Geometry check sheet. Reference: the model listing, model coordinates, mm. Coordinates: 2 decimals unless noted, no trailing zeros. Order: outer loops, then holes, each group sorted by start corner. A loop starts at its lowest first (then second) coordinate and runs counter-clockwise, first axis right, second up. Notation, with made-up numbers: (72.5, 73) - (78.5, 73) arc R14 cw to (78.5, 100) - close; hole circle Ø4 at (7.25, 14.25). An arc over 180 degrees is marked (long way). Put each result on its own line as item: value.
from build123d import *

# Parameters (mm, degrees)
SKETCH1_W                = 304
SKETCH1_H                = 304
BOSS_EXTRUDE1_DEPTH      = 2
SKETCH2_W                = 88
SKETCH2_H                = 15
CUT_EXTRUDE1_DEPTH       = 215.969765316
SKETCH7_W                = 50
SKETCH7_H                = 45
CUT_EXTRUDE2_DEPTH       = 2
FILLET1_R                = 2
F_7_0_7_DIAMETER_HOLE1_D = 7
M5_CLEARANCE_HOLE1_D     = 5.3


with BuildPart() as part:
    # Sketch1 → Boss-Extrude1 (new body)
    with BuildSketch(Plane(origin=(0, 0, 0), x_dir=(1, 0, 0), z_dir=(0, 1, 0))):
        Rectangle(SKETCH1_W, SKETCH1_H)
    extrude(amount=BOSS_EXTRUDE1_DEPTH)

    # Sketch2 → Cut-Extrude1 (cut, through all)
    with BuildSketch(Plane(origin=(0, 2, 0), x_dir=(1, 0, 0), z_dir=(0, 1, 0))):
        with Locations((0, -144.5)):
            Rectangle(SKETCH2_W, SKETCH2_H)
        with BuildLine():
            Line((-152, 100), (-138, 100))
            ThreePointArc((-138, 100), (-128, 110), (-138, 120))
            Line((-138, 120), (-152, 120))
            Line((-152, 120), (-152, 100))
        make_face()
        with BuildLine():
            Line((152, 100), (138, 100))
            ThreePointArc((138, 100), (128, 110), (138, 120))
            Line((138, 120), (152, 120))
            Line((152, 120), (152, 100))
        make_face()
    extrude(amount=-CUT_EXTRUDE1_DEPTH, mode=Mode.SUBTRACT)

    # Sketch7 → Cut-Extrude2 (cut)
    with BuildSketch(Plane.XZ):
        with Locations((0, 114.5)):
            Rectangle(SKETCH7_W, SKETCH7_H)
    extrude(amount=-CUT_EXTRUDE2_DEPTH, mode=Mode.SUBTRACT)

    # Fillet1
    fillet1_edges = [part.edges().sort_by_distance(p)[0] for p in [
        (44, 1, 152),
        (-44, 1, 152),
        (-44, 1, 137),
        (44, 1, 137),
        (-152, 1, -100),
        (-152, 1, -120),
        (152, 1, -120),
        (152, 1, -100),
        (25, 1, 92),
        (25, 1, 137),
        (-25, 1, 137),
        (-25, 1, 92),
        (-152, 1, -152),
        (152, 1, -152),
        (152, 1, 152),
        (-152, 1, 152),
    ]]
    fillet(fillet1_edges, radius=FILLET1_R)

    # Ø7.0 (7) Diameter Hole1 (through all)
    with Locations(Plane(origin=(0, 2, 0), x_dir=(1, 0, 0), z_dir=(0, 1, 0))):
        with Locations((0, -6)):
            Hole(F_7_0_7_DIAMETER_HOLE1_D / 2)

    # M5 Clearance Hole1 (through all)
    with Locations(Plane(origin=(0, 2, 0), x_dir=(1, 0, 0), z_dir=(0, 1, 0))):
        with Locations((-138, 138), (138, 138), (138, -138), (-138, -138), (0, 6)):
            Hole(M5_CLEARANCE_HOLE1_D / 2)


solid = part.part
Q1. Section check B-B on y = 1.55. State how many separate pieces and enclosed holes the cut face has, then the cut area to 3 significant figures.
Answer block:
separate pieces: 1
enclosed holes: 6
area: 87,800 mm^2
Q2. Section check A-A on z = 102.5. Record the boundary of the cut face in (x, y).
Answer block:
outline: (-152, 0) - (-25, 0) - (-25, 2) - (-152, 2) - close; (25, 0) - (152, 0) - (152, 2) - (25, 2) - close
Q3. Section check D-D on z = -110. Record the boundary of the cut face in (x, y).
Answer block:
outline: (-128, 0) - (128, 0) - (128, 2) - (-128, 2) - close
Q4. Depth check by flat-ended pin: pin 1 Ø5 at (x, z) = (-138, -138) entering from -Y. Enter the tip coordinate at first touch or a pass-through.
Answer block:
pin 1: passes through
Q5. Section check C-C on x = 131.5. Record the boundary of the cut face in (y, z), then the cut area to 3 significant figures.
Answer block:
outline: (0, -152) - (2, -152) - (2, -117.6) - (0, -117.6) - close; (0, -102.4) - (2, -102.4) - (2, 152) - (0, 152) - close
area: 578 mm^2
Q6. Draft check along X on faces 1 (the cylindrical face through (0.759, 0.986, 9.417)), 2 (the flat face through (-2, 0, -2)), 3 (the cylindrical face through (128, 1, -110)), 4 (the cylindrical face through (-128, 1, -110)). Enter one of: pulls with the +X half, pulls with the -X half, needs draft (parallel to the pull), parting line crosses it, or undercut.
Answer block:
face 1: undercut
face 2: needs draft
face 3: pulls with the +X half
face 4: pulls with the -X half
Q7. Thickness scan on L1, parallel to Z at x = 138, y = 1.1; L2, parallel to X at y = 1, z = -138; L3, parallel to X at y = 0.3, z = 95.5. Record the ranges inside material, lowest first. Write a range as [from, to].
Answer block:
L1: z = [-152, -140.65], [-135.35, -120], [-100, 135.35], [140.65, 152]
L2: x = [-152, -140.65], [-135.35, 135.35], [140.65, 152]
L3: x = [-152, -25], [25, 152]
